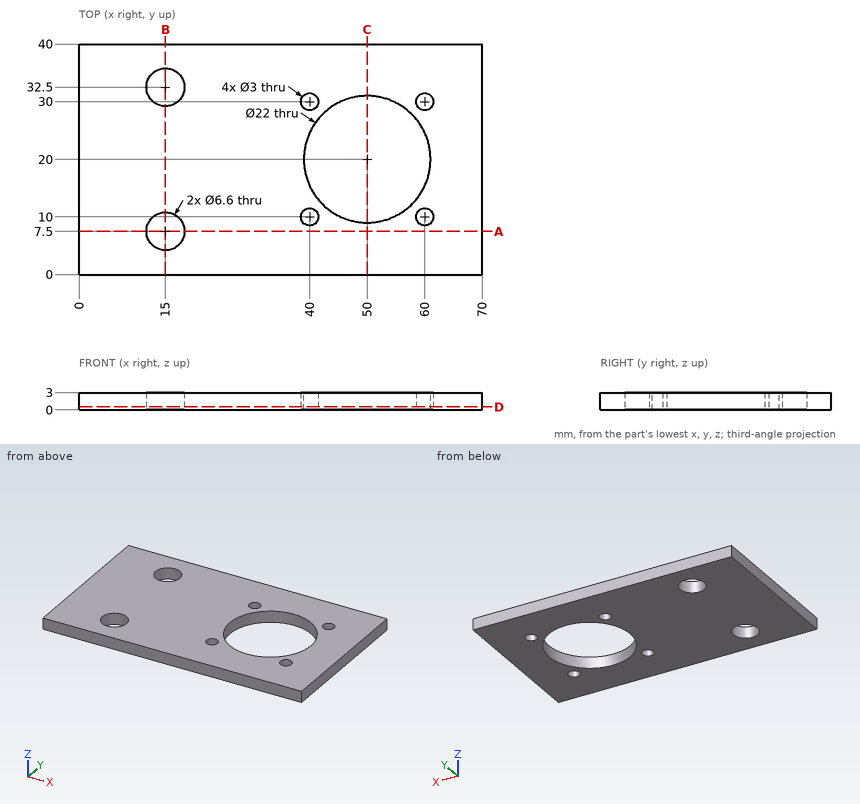
For this review, use the dimensioned drawing (mm, ordinates from the lowest corner) and the shaded views. Coordinates: 2 decimals unless noted, no trailing zeros. Write each loop counter-clockwise with the first axis right and the second up, starting at its lowest first coordinate (ties: lowest second). Pieces come first, ordered by that corner, then holes. Notation, with made-up numbers: (-12, 60.5) - (37, 60.5) arc R12 cw to (37, 77.5) - close; hole circle Ø4 at (42.25, 15.25). An arc over 180 degrees is marked (long way). Answer as a JSON object with one key per item and string values. Group by question number.
1. Add section C-C (x = 50). Give the boundary of the cut face in (y, z).
2. Clearance check with flat-ended pins moving along their axes: pin 1 Ø1 at (y, z) = (10, 2) entering from -X; pin 2 Ø2.5 at (x, y) = (60, 10) entering from +Z. State where each tip first meets the part, or that it passes through.
3. Add section A-A (y = 7.5). Give the boundary of the cut face in (x, z), plus the area to 3 significant figures.
4. Add section D-D (z = 0.5). Give the boundary of the cut face in (x, y).
5. To check wall thickness, follow probe 1 along Y at (x, z) = (15, 1); probe 2 along Y at (x, z) = (50, 1.6); probe 3 along Y at (x, z) = (40, 0.75). State the ranges of each line that lie inside material, in increasing order.
6. Add section B-B (x = 15). Give the boundary of the cut face in (y, z), plus the area to 3 significant figures.
Findings:
{
 "1": {"outline": "(0, 0) - (9, 0) - (9, 3) - (0, 3) - close; (31, 0) - (40, 0) - (40, 3) - (31, 3) - close"},
 "2": {"pin 1": "x = 0", "pin 2": "through"},
 "3": {"outline": "(0, 0) - (11.7, 0) - (11.7, 3) - (0, 3) - close; (18.3, 0) - (70, 0) - (70, 3) - (18.3, 3) - close", "area": "190 mm²"},
 "4": {"outline": "(0, 0) - (70, 0) - (70, 40) - (0, 40) - close; hole circle Ø6.6 at (15, 7.5); hole circle Ø6.6 at (15, 32.5); hole circle Ø3 at (40, 10); hole circle Ø3 at (40, 30); hole circle Ø22 at (50, 20); hole circle Ø3 at (60, 10); hole circle Ø3 at (60, 30)"},
 "5": {"probe 1": "0 to 4.2, 10.8 to 29.2, 35.8 to 40", "probe 2": "0 to 9, 31 to 40", "probe 3": "0 to 8.5, 11.5 to 15.42, 24.58 to 28.5, 31.5 to 40"},
 "6": {"outline": "(0, 0) - (4.2, 0) - (4.2, 3) - (0, 3) - close; (10.8, 0) - (29.2, 0) - (29.2, 3) - (10.8, 3) - close; (35.8, 0) - (40, 0) - (40, 3) - (35.8, 3) - close", "area": "80.4 mm²"}
}
